The figure shows three views and two pictorial views of one solid part (mm, origin at its lowest corner). Answer the questions. Give positions to 0.01 mm unless a question says otherwise; leave off trailing zeros. Loops run counter-clockwise (first coordinate to the right, second up) from the corner with the lowest first, then second, coordinate; pieces in that order, holes last. Notation, with made-up numbers: (-16.75, 79.25) - (11.25, 79.25) arc R7 ccw to (11.25, 87.25) - close; hole circle Ø9 at (21, 23.5). An arc over 180 degrees is marked (long way). Write each question's results on one line, items separated by ' | '.
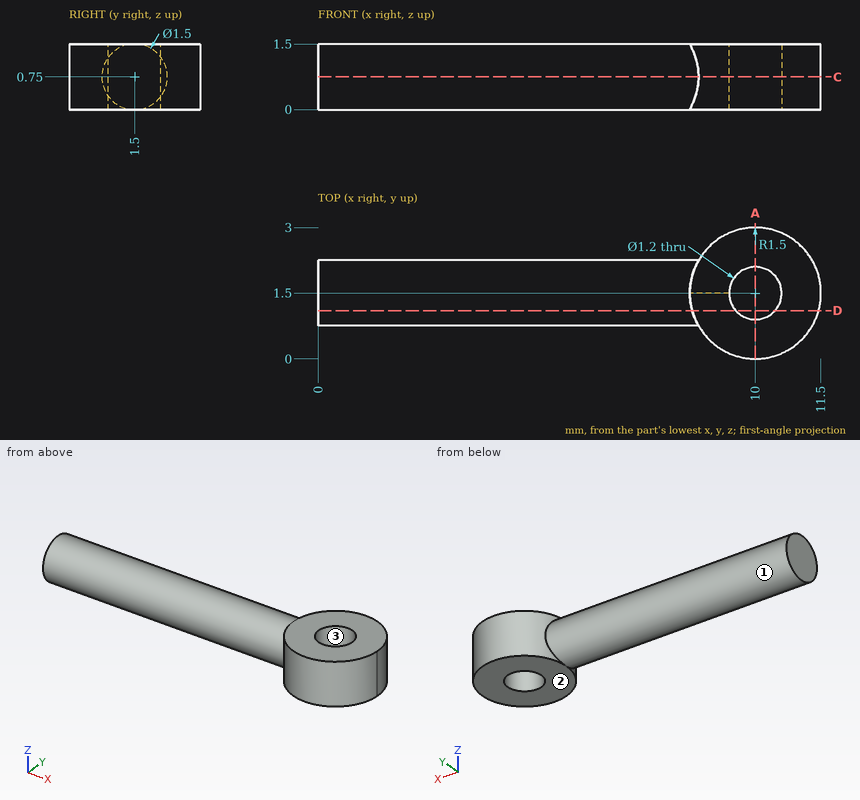
Item 1: A cutting plane is placed at D-D, the plane y = 1.1. Determine the outline of the cut face in (x, z), plus the area to 3 significant figures.
Values found:
outline: (0, 0.12) - (8.55, 0.12) - (8.55, 0) - (9.55, 0) - (9.55, 1.5) - (8.55, 1.5) - (8.55, 1.38) - (0, 1.38) - close; (10.45, 0) - (11.45, 0) - (11.45, 1.5) - (10.45, 1.5) - close | area: 13.8 mm²
Item 2: Find the intervals of material crossed by line 1 along Y through (x, z) = (10, 0.9); line 2 along X through (y, z) = (1.95, 1.1); line 3 along X through (y, z) = (2, 0.5), in increasing order. Write a range as [from, to].
Values found:
line 1: y = [0, 0.9], [2.1, 3] | line 2: x = [0, 9.6], [10.4, 11.43] | line 3: x = [0, 9.67], [10.33, 11.41]
Item 3: A flat-ended cylindrical pin translates along its axis: P1, Ø1, axis at x = 10, y = 1.5, coming from the +Z side. Find the tip coordinate at first contact, or state that the pin passes through.
Values found:
P1: passes through
Item 4: For a pull along Y with two mould halves and no side action, classify the marked faces 1, 2 and 3 as released by +Y, released by -Y, zero draft, split by the parting line, or undercut.
Values found:
face 1: split by the parting line | face 2: zero draft | face 3: undercut
Item 5: A cutting plane is placed at A-A, the plane x = 10. Determine the outline of the cut face in (y, z).
Values found:
outline: (0, 0) - (0.9, 0) - (0.9, 1.5) - (0, 1.5) - close; (2.1, 0) - (3, 0) - (3, 1.5) - (2.1, 1.5) - close
Item 6: A cutting plane is placed at C-C, the plane z = 0.75. Determine the outline of the cut face in (x, y).
Values found:
outline: (0, 0.75) - (8.7, 0.75) arc R1.5 ccw (long way) to (8.7, 2.25) - (0, 2.25) - close; hole circle Ø1.2 at (10, 1.5)
